Input: part model. Units: mm. Frame: model coordinates. A direction names the side the tool comes from. Coordinates: 2 decimals unless noted, no trailing zeros. Loops run counter-clockwise (first coordinate to the right, second up) from the corner with the lowest first, then second, coordinate; pieces in that order, holes last. Notation, with made-up numbers: (45, 74.25) -> (49, 74.25) arc R14 ccw to (49, 89.25) -> close; hole circle Ø3 at (9.25, -27.5). An arc over 180 degrees is marked (long way). Put each result on its own line as item: value. Start each with the question number.
1) Pull-direction query (X, two-part tool) for faces 5 (the flat face through (0, 66, 10)), 6 (the flat face through (9.01, 59.26, 10.14)), 7 (the flat face through (4, 66, 20)); classes: pulls with the +X half, pulls with the -X half, needs draft (parallel to the pull), parting line crosses it, or undercut.
2) Contact query for flat-ended pins moving along their axis: P1, Ø10, axis at x = 16.5, y = 34.5, coming from the +Z side; P2, Ø1.1, axis at x = 52, y = -2.5, coming from the +Z side; P3, Ø1, axis at x = 15, z = 15, coming from the -Y side. Output: stop coordinate, or through.
3) Set-up query: faces 1 (the cylindrical face through (50.25, 127.77, 14)), 2 (the flat face through (80.99, 59.26, 10.14)), 3 (the flat face through (80, 81, 10)), 4 (the flat face through (4, 66, 0)). Return all of +Z, -Z, +X, -X, +Y, -Y with unobstructed straight access to the full face (end or side cutting, diameter ignored); none if empty.
4) Cut plane A-A (x = 29.5). Return the cut outline in (y, z), plus the area to 3 significant figures.
5) Material intervals for L1, parallel to X at y = 56.5, z = 10.25; L2, parallel to Y at x = 39.5, z = 17; L3, parallel to X at y = 78.5, z = 4.5, sorted ascending.
6) Cut plane B-B (y = 27). Return the cut outline in (x, z), plus the area to 3 significant figures.
7) Cut plane C-C (z = 10.25). Return the cut outline in (x, y).
Autodesk Inventor part; units mm, degrees
ref_plane "YZ Plane" through (0, 0, 0) normal (1, 0, 0) x (0, 1, 0)
ref_plane "XZ Plane" through (0, 0, 0) normal (0, 1, 0) x (-1, 0, 0)
ref_plane "XY Plane" through (0, 0, 0) normal (0, 0, 1) x (1, 0, 0)
sketch "Sketch1" plane through (0, 0, 0) normal (0, 0, 1) x (1, 0, 0)
  line L0 (0, 0) -> (90, 0)
  line L1 (90, 0) -> (90, 130)
  line L2 (90, 130) -> (0, 130)
  line L3 (0, 130) -> (0, 0)
  line L4 (10, 20) -> (80, 20)
  line L5 (80, 20) -> (80, 110)
  line L6 (80, 110) -> (10, 110)
  line L7 (10, 110) -> (10, 20)
  dimension "d0" = 90
  dimension "d1" = 130
  dimension "d2" = 70
  dimension "d3" = 90
  dimension "d16" = 20
  dimension "d17" = 20
  dimension "d18" = 10
extrude "Extrusion1" add sketch "Sketch1" along normal blind 20
sketch "Sketch2" plane through (10, 20, 0) normal (1, 0, 0) x (0, 0, -1)
  line L0 (0, 90) -> (0, 0)
  line L1 (0, 42.1132) -> (-20, 30.5662)
  line L2 (-20, 110) -> (-20, -20)
  line L3 (0, 42.1132) -> (23.094, 42.1132) construction
  line L4 (-20, 30.5662) -> (-20, 33.5662)
  line L5 (-20, 33.5662) -> (0, 45.1132)
  line L6 (0, 42.1132) -> (0, 45.1132)
  point P0 (-20, 0)
  point P1 (0, -20)
  dimension "d6" = 210
  dimension "d7" = 3
  dimension "d8" = 26.4711
extrude "Extrusion2" cut sketch "Sketch2" against normal blind 2
sketch "Sketch3" plane through (80, 20, 0) normal (-1, 0, 0) x (0, 0, 1)
  line L0 (0, 0) -> (0, 90)
  line L1 (20, 90) -> (20, 0)
  line L2 (0, 42.1132) -> (20, 30.5662)
  line L3 (0, 42.1132) -> (23.094, 42.1132) construction
  line L4 (20, 30.5662) -> (20, 33.5662)
  line L5 (20, 33.5662) -> (0, 45.1132)
  line L6 (0, 42.1132) -> (0, 45.1132)
  point P0 (0, -20)
  dimension "d11" = 30
  dimension "d12" = 3
  dimension "d13" = 26.4711
extrude "Extrusion3" cut sketch "Sketch3" against normal blind 2
sketch "Sketch4" plane through (0, 0, 0) normal (0, -1, 0) x (1, 0, 0)
  line L0 (0, 0) -> (90, 0)
  line L1 (90, 0) -> (90, 20)
  line L2 (0, 20) -> (90, 20)
  line L3 (0, 0) -> (0, 20)
  line L4 (55, 3) -> (35, 3)
  line L5 (35, 3) -> (35, 17)
  line L6 (35, 17) -> (55, 17)
  line L7 (55, 17) -> (55, 3)
  line L8 (53.2053, 7.41) -> (53.87, 5.3643)
  line L9 (53.87, 5.3643) -> (52.1298, 4.1)
  line L10 (52.1298, 4.1) -> (50.3897, 5.3643)
  line L11 (50.3897, 5.3643) -> (51.0543, 7.41)
  line L12 (51.0543, 7.41) -> (53.2053, 7.41)
  line L13 (38.9443, 7.41) -> (39.609, 5.3643)
  line L14 (39.609, 5.3643) -> (37.8689, 4.1)
  line L15 (37.8689, 4.1) -> (36.1287, 5.3643)
  line L16 (36.1287, 5.3643) -> (36.7934, 7.41)
  line L17 (36.7934, 7.41) -> (38.9443, 7.41)
  line L18 (38.9447, 15.55) -> (39.6093, 13.5043)
  line L19 (39.6093, 13.5043) -> (37.8692, 12.24)
  line L20 (37.8692, 12.24) -> (36.129, 13.5043)
  line L21 (36.129, 13.5043) -> (36.7937, 15.55)
  line L22 (36.7937, 15.55) -> (38.9447, 15.55)
  line L23 (53.2053, 15.55) -> (53.87, 13.5043)
  line L24 (53.87, 13.5043) -> (52.1298, 12.24)
  line L25 (52.1298, 12.24) -> (50.3897, 13.5043)
  line L26 (50.3897, 13.5043) -> (51.0543, 15.55)
  line L27 (51.0543, 15.55) -> (53.2053, 15.55)
  point P0 (52.1298, 5.9297)
  point P1 (37.8689, 5.9297)
  point P2 (37.8692, 14.0697)
  point P3 (52.1298, 14.0697)
  dimension "d19" = 20
  dimension "d20" = 14
  dimension "d21" = 3
  dimension "d22" = 3
  dimension "d23" = 35
  dimension "d24" = 35
  dimension "d25" = 1.45
  dimension "d26" = 1.45
  dimension "d27" = 1.1
  dimension "d28" = 1.1
  dimension "d29" = 12.11
  dimension "d30" = 1.13
  dimension "d31" = 1.13
  dimension "d32" = 4.83
  dimension "d33" = 4.83
  dimension "d34" = 1.129
  dimension "d35" = 1.1287
extrude "Extrusion4" add sketch "Sketch4" along normal blind 4 contours L8 L9 L10 L11 L12 | L13 L14 L15 L16 L17 | L18 L19 L20 L21 L22 | L23 L24 L25 L26 L27
chamfer "Chamfer1" distance 0.5 angle 45 20 edges at (52.1298, -4, 15.55) (50.722, -4, 14.5272) (51.2597, -4, 12.8722) (52.9999, -4, 12.8722) (53.5377, -4, 14.5272) (52.1298, -4, 7.41) (53.5377, -4, 6.3872) (52.9999, -4, 4.7322) (51.2597, -4, 4.7322) (50.722, -4, 6.3872) (39.277, -4, 14.5272) (38.7393, -4, 12.8722) (36.9991, -4, 12.8722) (36.4613, -4, 14.5272) (37.8692, -4, 15.55) (37.8689, -4, 7.41) (39.2767, -4, 6.3872) (38.7389, -4, 4.7322) (36.9988, -4, 4.7322) (36.461, -4, 6.3872)
sketch "Sketch5" plane through (0, 130, 0) normal (0, 1, 0) x (1, 0, 0)
  line L0 (90, 0) -> (0, 0)
  line L1 (0, 0) -> (0, -20)
  line L2 (90, -20) -> (0, -20)
  line L3 (90, 0) -> (90, -20)
  line L4 (55, -17) -> (35, -17)
  line L5 (35, -17) -> (35, -3)
  line L6 (35, -3) -> (55, -3)
  line L7 (55, -3) -> (55, -17)
  line L8 (52.2861, -15.9) -> (50.4139, -14.8429)
  line L9 (50.4139, -14.8429) -> (50.8408, -12.7357)
  line L10 (50.8408, -12.7357) -> (52.9767, -12.4905)
  line L11 (52.9767, -12.4905) -> (53.87, -14.4461)
  line L12 (53.87, -14.4461) -> (52.2861, -15.9)
  line L13 (37.7119, -15.9) -> (36.128, -14.4461)
  line L14 (36.128, -14.4461) -> (37.0213, -12.4905)
  line L15 (37.0213, -12.4905) -> (39.1572, -12.7357)
  line L16 (39.1572, -12.7357) -> (39.5841, -14.8429)
  line L17 (39.5841, -14.8429) -> (37.7119, -15.9)
  line L18 (37.8674, -7.7585) -> (36.128, -6.4948)
  line L19 (36.128, -6.4948) -> (36.7924, -4.45)
  line L20 (36.7924, -4.45) -> (38.9424, -4.45)
  line L21 (38.9424, -4.45) -> (39.6068, -6.4948)
  line L22 (39.6068, -6.4948) -> (37.8674, -7.7585)
  line L23 (52.1306, -7.7585) -> (50.3912, -6.4948)
  line L24 (50.3912, -6.4948) -> (51.0556, -4.45)
  line L25 (51.0556, -4.45) -> (53.2056, -4.45)
  line L26 (53.2056, -4.45) -> (53.87, -6.4948)
  line L27 (53.87, -6.4948) -> (52.1306, -7.7585)
  circle A0 centre (52.0775, -14.083) radius 1.8289
  circle A1 centre (37.9205, -14.083) radius 1.8289
  circle A2 centre (37.8674, -5.9296) radius 1.8289
  circle A3 centre (52.1306, -5.9296) radius 1.8289
  dimension "d41" = 20
  dimension "d42" = 14
  dimension "d43" = 3
  dimension "d44" = 3
  dimension "d45" = 35
  dimension "d46" = 35
  dimension "d62" = 2.15
  dimension "d63" = 2.15
  dimension "d64" = 2.15
  dimension "d65" = 2.15
  dimension "d66" = 1.13
  dimension "d67" = 1.13
  dimension "d68" = 1.128
  dimension "d69" = 1.1
  dimension "d70" = 1.1
  dimension "d71" = 1.45
  dimension "d72" = 1.45
  dimension "d73" = 1.128
extrude "Extrusion5" cut sketch "Sketch5" against normal blind 4 contours A0 L8 | L8 L9 L10 L11 L12 | L12 A0 | A0 L9 | L11 A0 | A0 L10 | A1 L13 | L13 L14 L15 L16 L17 | L17 A1 | A1 L14 | L16 A1 | A1 L15 | A2 L18 | L18 L19 L20 L21 L22 | L22 A2 | A2 L19 | L21 A2 | A2 L20 | A3 L23 | L23 L24 L25 L26 L27 | L27 A3 | A3 L24 | L26 A3 | A3 L25
chamfer "Chamfer2" distance 0.5 angle 45 4 edges at (50.2486, 130, 14.083) (36.0916, 130, 14.083) (36.0385, 130, 5.9296) (50.3017, 130, 5.9296)
properties part number "Frame V2"
Results found:
1. face 5: pulls with the -X half
1. face 6: undercut
1. face 7: needs draft
2. P1: passes through
2. P2: stops at z = 15.55
2. P3: stops at y = 0
3. face 1: +Y
3. face 2: none
3. face 3: +Z, -Z
3. face 4: -Z, +X, -X, +Y, -Y
4. outline: (0, 0) -> (20, 0) -> (20, 20) -> (0, 20) -> close; (110, 0) -> (130, 0) -> (130, 20) -> (110, 20) -> close
4. area: 800 mm2
5. L1: x = 0 to 8, 82 to 90
5. L2: y = 0 to 20, 110 to 130
5. L3: x = 0 to 10, 80 to 90
6. outline: (0, 0) -> (10, 0) -> (10, 20) -> (0, 20) -> close; (80, 0) -> (90, 0) -> (90, 20) -> (80, 20) -> close
6. area: 400 mm2
7. outline: (0, 0) -> (90, 0) -> (90, 130) -> (0, 130) -> close; hole (8, 56.2) -> (10, 56.2) -> (10, 20) -> (80, 20) -> (80, 56.2) -> (82, 56.2) -> (82, 59.2) -> (80, 59.2) -> (80, 110) -> (10, 110) -> (10, 59.2) -> (8, 59.2) -> close
